Work out the finished part from the listing and answer in its coordinate system (mm). Face numbers are marked on the shaded views. A direction names the side the tool comes from. Coordinates: 2 decimals unless noted, no trailing zeros. Order: outer loops, then holes, each group sorted by start corner. A loop starts at its lowest first (then second) coordinate and runs counter-clockwise, first axis right, second up. Notation, with made-up numbers: (40, 28.5) - (66, 28.5) arc R31 cw to (66, 57.5) - close; hole circle Ø7 at (85, 41). An arc over 180 degrees is marked (long way). Answer as a JSON object with one key per item and string values. Group by question number.
1) A tool of negligible diameter and unlimited length cuts with its end or side. For the marked faces 1 and 2, from which of +Z, -Z, +X, -X, +Y, -Y can it reach the whole face along a straight path? Write none if from no direction.
2) Section B-B (z = 76.5) is taken. Give the vertices of the cut face in (x, y).
3) Each of these flat-tipped pins is pushed along its axis until it touches: P1, Ø2, axis at x = 14.5, z = 57, coming from the +Y side; P2, Ø1, axis at x = -32, y = -27.5, coming from the -Z side; P3, Ø1.5, axis at x = 31.5, z = 21.5, coming from the -Y side. Where does it stop, or does it pass through?
4) The mould has two halves that part along X. Classify the marked faces 3 and 4: released by +X, released by -X, zero draft, split by the parting line, or undercut.
5) Find the intervals of material crossed by line 1 along Y through (x, z) = (0, 19.5); line 2 along X through (y, z) = (-11, 96), in increasing order.
6) Section A-A (z = 56) is taken. Give the vertices of the cut face in (x, y).
from build123d import *

# Parameters (mm, degrees)
F2_R = 5.08
F3_R = 5.08
F4_T = -2


with BuildPart() as f1:
    # F0 (on Front) → F1 (revolve)
    with BuildSketch(Plane.XZ):
        Polygon((0, 150), (0, 0), (45, 0), (45, 65.276236894), (31.6620995219, 108.2541429718), (10, 129.0087435294), (10, 150), align=None)
    revolve(axis=Axis((0, 0, 75), (0, 0, -1)))

    # F2
    f2_edges = [f1.edges().sort_by_distance(p)[0] for p in [
        (-45, 0, 0),
        (-45, 0, 65.276237),
        (45, 0, 32.638118),
    ]]
    fillet(f2_edges, radius=F2_R)

    # F3
    f3_edges = [f1.edges().sort_by_distance(p)[0] for p in [
        (-31.6621, 0, 108.254143),
    ]]
    fillet(f3_edges, radius=F3_R)

    # F4
    f4_openings = [f1.faces().sort_by_distance(p)[0] for p in [
        (0, 0, 150),
    ]]
    offset(amount=F4_T, openings=f4_openings, kind=Kind.INTERSECTION)


solid = f1.part
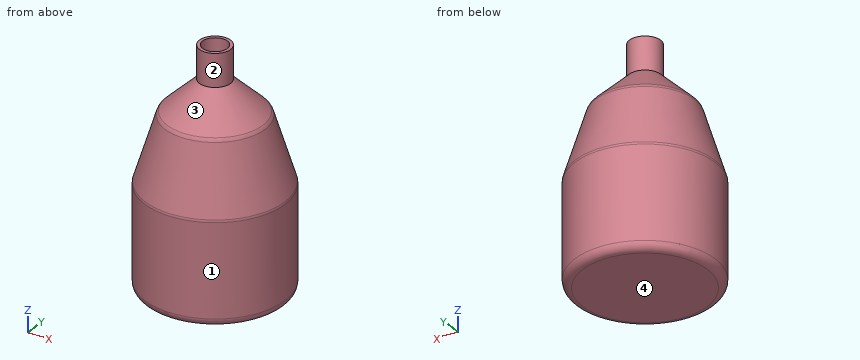
Report:
{
 "1": {"face 1": "+Z, -Z", "face 2": "+Z"},
 "2": {"outline": "circle Ø83.03 at (0, 0); hole circle Ø78.85 at (0, 0)"},
 "3": {"P1": "stops at y = 42.93", "P2": "stops at z = 0.32", "P3": "stops at y = -32.85"},
 "4": {"face 3": "split by the parting line", "face 4": "zero draft"},
 "5": {"line 1": "y = -45 to -43, 43 to 45", "line 2": "x = -33.72 to -31.51, 31.51 to 33.72"},
 "6": {"outline": "circle Ø90 at (0, 0); hole circle Ø86 at (0, 0)"}
}
